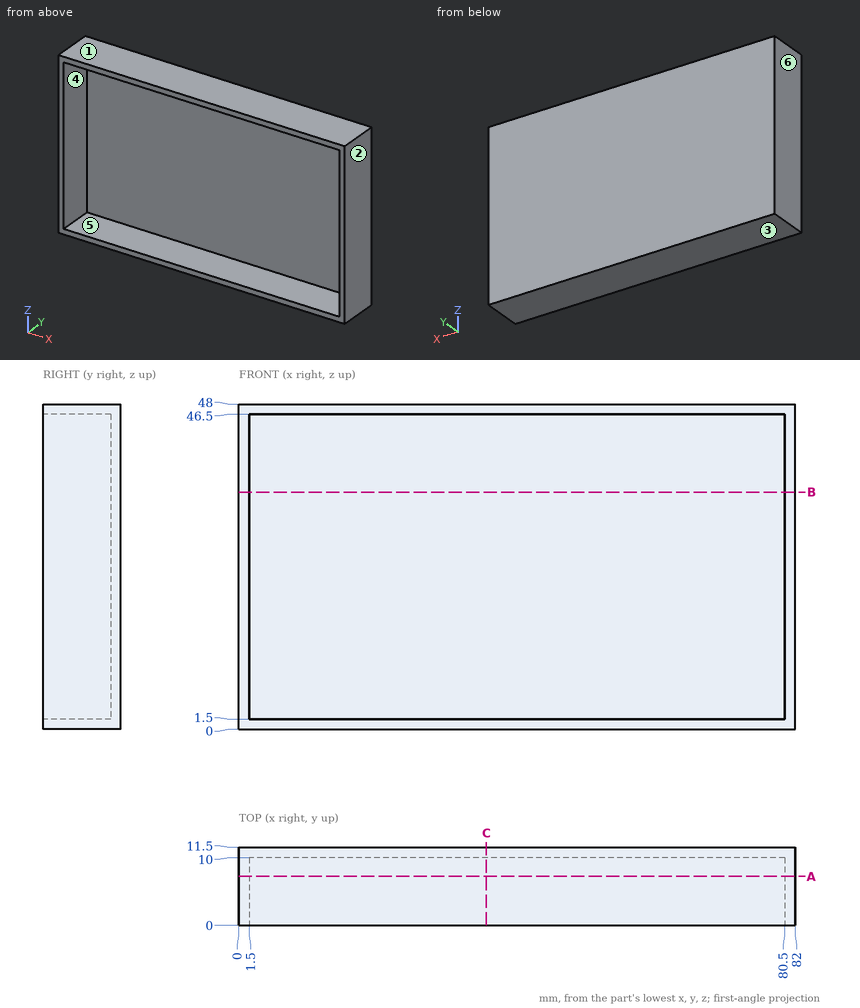
The figure shows three views and two pictorial views of one solid part (mm, origin at its lowest corner). Answer the questions. A direction names the side the tool comes from. Round coordinates to 2 decimals unless told otherwise and drop trailing zeros. Order: outer loops, then holes, each group sorted by start corner. A loop starts at its lowest first (then second) coordinate and runs counter-clockwise, first axis right, second up. Notation, with made-up numbers: (27, 69.5) -> (83, 69.5) arc R30 ccw to (83, 105.5) -> close; hole circle Ø9 at (42.5, 31). An arc over 180 degrees is marked (long way). Put each result on its own line as item: value.
Q1. Determine the mould class of the marked faces 1, 2, 3 and 4 for opening direction Z: pulls with the +Z half, pulls with the -Z half, needs draft (parallel to the pull), parting line crosses it, or undercut.
Results list:
face 1: pulls with the +Z half
face 2: needs draft
face 3: pulls with the -Z half
face 4: undercut
Q2. Section C-C, the plane x = 36.5 is taken. Write down the section's boundary in (y, z).
Results list:
outline: (0, 0) -> (11.5, 0) -> (11.5, 48) -> (0, 48) -> (0, 46.5) -> (10, 46.5) -> (10, 1.5) -> (0, 1.5) -> close
Q3. Each of these flat-tipped pins is pushed along its axis until it touches: P1, Ø3, axis at x = 40.5, y = 6, coming from the -Z side; P2, Ø13.5, axis at x = 52, z = 21, coming from the -Y side. Where does it stop, or does it pass through?
Results list:
P1: z = 0
P2: y = 10
Q4. Section B-B, the plane z = 35 is taken. Write down the section's boundary in (x, y), and give its area (3 significant figures).
Results list:
outline: (0, 0) -> (1.5, 0) -> (1.5, 10) -> (80.5, 10) -> (80.5, 0) -> (82, 0) -> (82, 11.5) -> (0, 11.5) -> close
area: 153 mm^2
Q5. Section A-A, the plane y = 7.25 is taken. Write down the section's boundary in (x, z).
Results list:
outline: (0, 0) -> (82, 0) -> (82, 48) -> (0, 48) -> close; hole (1.5, 1.5) -> (80.5, 1.5) -> (80.5, 46.5) -> (1.5, 46.5) -> close
Q6. Which of the six approach directions +Z, -Z, +X, -X, +Y, -Y give full straight-line access (tool end or side, diameter ignored) to the marked faces 5 and 6?
Results list:
face 5: -Y
face 6: +Z, -Z, -X, +Y, -Y
Q7. Consider line 1 along Z through (x, y) = (78, 3.75); line 2 along X through (y, z) = (5, 40); line 3 along Y through (x, z) = (28.5, 10). Determine where each line is inside the solid, lowest interval first.
Results list:
line 1: 0 to 1.5, 46.5 to 48
line 2: 0 to 1.5, 80.5 to 82
line 3: 10 to 11.5
